The listing builds one solid part. Answer for the finished solid, in the listing's coordinates (mm). Coordinates: 2 decimals unless noted, no trailing zeros. Order: outer loops, then holes, each group sorted by start corner. A loop starts at its lowest first (then second) coordinate and runs counter-clockwise, first axis right, second up. Notation, with made-up numbers: (83.5, -19) -> (133.5, -19) arc R34 ccw to (133.5, 19) -> close; hole circle Ø9 at (2.25, 80.5). An arc over 180 degrees is marked (long way). Return JSON: item names as keys, results as strings.
from build123d import *

# Parameters (mm, degrees)
F0_W     = 220
F0_H     = 315
F1_DEPTH = 5
F2_R     = 25
F3_DEPTH = 25
F4_R     = 5


with BuildPart() as f1:
    # F0 (on Front) → F1 (new body)
    with BuildSketch(Plane.XZ):
        Rectangle(F0_W, F0_H)
    extrude(amount=F1_DEPTH)

    # F2 (on face) → F3 (cut)
    with BuildSketch(Plane.XZ.offset(5)):
        with Locations((110, 0)):
            Circle(F2_R)
    extrude(amount=-F3_DEPTH, mode=Mode.SUBTRACT)

    # F4
    f4_edges = [f1.edges().sort_by_distance(p)[0] for p in [
        (110, -2.5, -25),
        (110, -2.5, 25),
        (110, -2.5, 157.5),
        (-110, -2.5, 157.5),
        (-110, -2.5, -157.5),
        (110, -2.5, -157.5),
    ]]
    fillet(f4_edges, radius=F4_R)


solid = f1.part
1. Determine the mould class of faces 1 (the face through (85, -3, 0)), 2 (the face through (-2, -5, 2)) for opening direction Z: pulls with the +Z half, pulls with the -Z half, needs draft (parallel to the pull), parting line crosses it, or undercut.
Answer block:
{"face 1": "undercut", "face 2": "needs draft"}
2. The part is cut by section A-A on z = -15.5. Give the vertices of the cut face in (x, y), and give its area (3 significant figures).
Answer block:
{"outline": "(-110, -5) -> (90.38, -5) -> (90.38, 0) -> (-110, 0) -> close", "area": "1,000 mm2"}
3. Consider line 1 (Z direction, x = 93, y = -1.7); line 2 (X direction, y = -4.4, z = 11.5); line 3 (X direction, y = -3.15, z = 4). Determine where each line is inside the solid, lowest interval first. Write a range as from..to.
Answer block:
{"line 1": "z = -157.5..-18.33, 18.33..157.5", "line 2": "x = -110..87.8", "line 3": "x = -110..85.32"}
